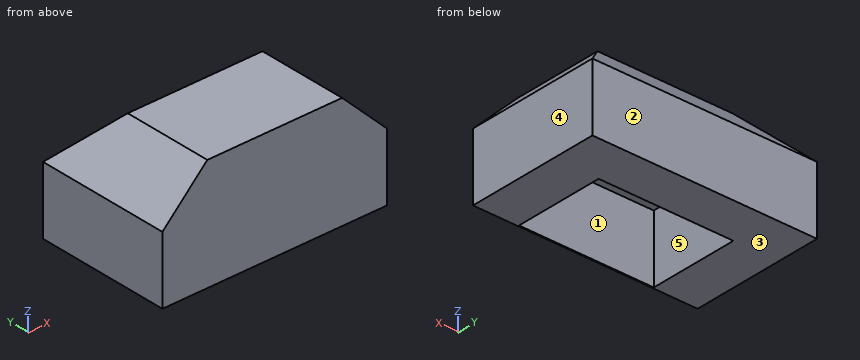
```python
from build123d import *

# Parameters (mm, degrees)
F0_W     = 10
F0_H     = 6
F2_DEPTH = 5
F1_W     = 6
F1_H     = 4
F3_DEPTH = 3
F4_SIZE  = 2


with BuildPart() as f2:
    # F0 (on Top) → F2 (new body)
    with BuildSketch(Plane.XY):
        with Locations((-22.542964, 15.566407)):
            Rectangle(F0_W, F0_H)
    extrude(amount=F2_DEPTH)

    # F1 (on face) → F3 (cut)
    with BuildSketch(Plane.XY):
        with Locations((-22.542964, 14.620967)):
            Rectangle(F1_W, F1_H)
    extrude(amount=F3_DEPTH, mode=Mode.SUBTRACT)

    # F4
    f4_edges = [f2.edges().sort_by_distance(p)[0] for p in [
        (-27.542964, 15.566407, 5),
        (-22.542964, 18.566407, 5),
        (-17.542964, 15.566407, 5),
    ]]
    chamfer(f4_edges, length=F4_SIZE)


solid = f2.part
```
Verification items for the finished model (mm, model axes). Face numbers are marked on the shaded views. A direction names the side the tool comes from. Round coordinates to 2 decimals unless told otherwise and drop trailing zeros. Order: outer loops, then holes, each group sorted by start corner. A loop starts at its lowest first (then second) coordinate and runs counter-clockwise, first axis right, second up.
1) Cross-section at B-B, the plane x = -25.25. Record the cut outline in (y, z), plus the area to 3 significant figures.
Geometry says:
outline: (12.57, 0) - (12.62, 0) - (12.62, 3) - (16.62, 3) - (16.62, 0) - (18.57, 0) - (18.57, 3) - (16.57, 5) - (12.57, 5) - close
area: 16.0 mm2
2) Depth check by flat-ended pin: pin 1 (3 mm diameter, centred on x = -24, y = 15, fed in from -Z). Enter the tip coordinate at first touch or a pass-through.
Geometry says:
pin 1: stops at z = 3
3) Cross-section at C-C, the plane y = 13.8. Record the cut outline in (x, z).
Geometry says:
outline: (-27.54, 0) - (-25.54, 0) - (-25.54, 3) - (-19.54, 3) - (-19.54, 0) - (-17.54, 0) - (-17.54, 3) - (-19.54, 5) - (-25.54, 5) - (-27.54, 3) - close
4) Tool access check on the marked faces 4 and 5. Record the directions out of +Z, -Z, +X, -X, +Y, -Y that give a thin tool (end or side, any length) a straight path to the whole face; none if there is none.
Geometry says:
face 4: +Z, -Z, +X, +Y, -Y
face 5: -Z
5) Cross-section at A-A, the plane z = 2.5. Record the cut outline in (x, y).
Geometry says:
outline: (-27.54, 12.57) - (-17.54, 12.57) - (-17.54, 18.57) - (-27.54, 18.57) - close; hole (-25.54, 12.62) - (-19.54, 12.62) - (-19.54, 16.62) - (-25.54, 16.62) - close
6) Cross-section at D-D, the plane x = -18.25. Record the cut outline in (y, z).
Geometry says:
outline: (12.57, 0) - (18.57, 0) - (18.57, 3) - (17.86, 3.71) - (12.57, 3.71) - close
7) Draft check along Y on the marked faces 1, 2 and 3. Enter one of: +Y half, -Y half, draft (parallel to the pull), parting line (faces both ways), or undercut.
Geometry says:
face 1: undercut
face 2: +Y half
face 3: draft
8) Material ranges on line 1 (X direction, y = 13.35, z = 2.3); line 2 (Z direction, x = -25.25, y = 15.7); line 3 (Y direction, x = -22, z = 4), recorded low to high.
Geometry says:
line 1: x = -27.54 to -25.54, -19.54 to -17.54
line 2: z = 3 to 5
line 3: y = 12.57 to 17.57
